The listing builds one solid part. Answer for the finished solid, in the listing's coordinates (mm). Coordinates: 2 decimals unless noted, no trailing zeros. Loops run counter-clockwise (first coordinate to the right, second up) from the corner with the lowest first, then second, coordinate; pieces in that order, holes last. Notation, with made-up numbers: M 76,59 L 119,59 A19 cw 119,76 Z; hole C -16.5,59.5 d2. An arc over 180 degrees is marked long. Answer as a JSON object with one key per item and string values. Group by question number.
1. A cutting plane is placed at A-A on z = 29. Give the vertices of the cut face in (x, y) (3 decimals), and give its area (3 significant figures).
2. Given pin 1 (2 mm diameter, centred on y = 92.5, z = -59.5, fed in from -X); pin 2 (1.5 mm diameter, centred on x = 2.5, z = 53.5, fed in from -Y); pin 3 (1.5 mm diameter, centred on x = 1, y = -13, fed in from +Z), each flat-ended and moving along its own axis, determine where each tip first touches the part or whether it passes through.
3. Straight lines are drawn through the part: L1, parallel to Y at x = 1.05, z = 29; L2, parallel to Z at x = 1.4, y = 48; L3, parallel to Z at x = 0.4, y = 32.5. For each, find the intervals that lie inside material, in ascending order.
4. A cutting plane is placed at D-D on x = 2.15. Give the vertices of the cut face in (y, z) (3 decimals).
5. A cutting plane is placed at B-B on y = 13. Give the vertices of the cut face in (x, z) (3 decimals), and give its area (4 significant figures).
6. A cutting plane is placed at C-C on z = 0. Give the vertices of the cut face in (x, y) (3 decimals).
from build123d import *

# Parameters (mm, degrees)
SKETCH1_R           = 127
SKETCH1_R_2         = 3.175
BOSS_EXTRUDE1_DEPTH = 3.175


with BuildPart() as part:
    # Sketch1 → Boss-Extrude1 (new body)
    with BuildSketch(Plane(origin=(0, 0, 0), x_dir=(0, 0, -1), z_dir=(1, 0, 0))):
        Circle(SKETCH1_R)
        with Locations((-29, -50.229473419)):
            Circle(SKETCH1_R_2, mode=Mode.SUBTRACT)
        with Locations((29, -50.229473419)):
            Circle(SKETCH1_R_2, mode=Mode.SUBTRACT)
        with Locations((-58, 0)):
            Circle(SKETCH1_R_2, mode=Mode.SUBTRACT)
        with Locations((-29, 50.229473419)):
            Circle(SKETCH1_R_2, mode=Mode.SUBTRACT)
        with BuildLine():
            ThreePointArc((26, 45.033320997), (45.033320997, 26), (52, 0))
            ThreePointArc((52, 0), (-45.033320997, -26), (26, 45.033320997))
        make_face(mode=Mode.SUBTRACT)
        with Locations((58, 0)):
            Circle(SKETCH1_R_2, mode=Mode.SUBTRACT)
        with Locations((29, 50.229473419)):
            Circle(SKETCH1_R_2, mode=Mode.SUBTRACT)
    extrude(amount=BOSS_EXTRUDE1_DEPTH)


solid = part.part
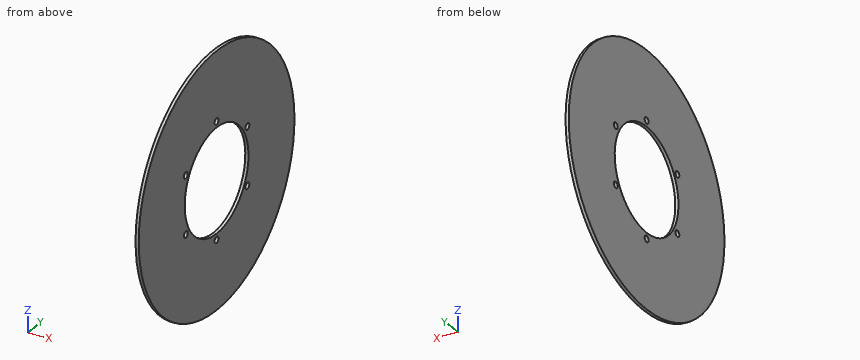
From the geometry:
{
 "1": {"outline": "M 0,-123.645 L 3.175,-123.645 L 3.175,-53.404 L 0,-53.404 Z; M 0,-47.054 L 3.175,-47.054 L 3.175,-43.162 L 0,-43.162 Z; M 0,43.162 L 3.175,43.162 L 3.175,47.054 L 0,47.054 Z; M 0,53.404 L 3.175,53.404 L 3.175,123.645 L 0,123.645 Z", "area": "471 mm²"},
 "2": {"pin 1": "stops at x = 0", "pin 2": "stops at y = -115.53", "pin 3": "stops at z = 126.41"},
 "3": {"L1": "y = -123.64 to -53.4, -47.05 to -43.16, 43.16 to 47.05, 53.4 to 123.64", "L2": "z = -117.58 to -31.26, -26.74 to -20, 20 to 26.74, 31.26 to 117.58", "L3": "z = -122.77 to -40.59, 40.59 to 122.77"},
 "4": {"outline": "C 0,0 d254; hole C -50.229,-29 d6.35; hole C -50.229,29 d6.35; hole C 0,0 d104; hole C 0,-58 d6.35; hole C 0,58 d6.35; hole C 50.229,-29 d6.35; hole C 50.229,29 d6.35"},
 "5": {"outline": "M 0,-126.333 L 3.175,-126.333 L 3.175,-50.349 L 0,-50.349 Z; M 0,50.349 L 3.175,50.349 L 3.175,126.333 L 0,126.333 Z", "area": "482.5 mm²"},
 "6": {"outline": "M 0,-127 L 3.175,-127 L 3.175,-52 L 0,-52 Z; M 0,52 L 3.175,52 L 3.175,127 L 0,127 Z"}
}
